Answer from the drawing. Dimensions are ordinates in mm from the lowest x, y and z of the part. Coordinates: 2 decimals unless noted, no trailing zeros. Order: outer loops, then holes, each group sorted by start corner. A loop starts at its lowest first (then second) coordinate and runs counter-clockwise, first axis right, second up. Notation, with made-up numbers: (15.25, -26.5) -> (25.25, -26.5) arc R17 ccw to (25.25, 1.5) -> close; hole circle Ø1 at (75, -26.5). An arc over 180 degrees is marked (long way). Answer as a JSON object with one key per item and string values. Group by question number.
1) Section B-B on x = 10.25 is taken. Determine the outline of the cut face in (y, z).
2) Section A-A on y = 31.75 is taken. Determine the outline of the cut face in (x, z).
3) Consider L1, parallel to X at y = 31.75, z = 1.25; L2, parallel to Y at x = 12.7, z = 0.6; L3, parallel to Y at x = 6.25, z = 0.8. Determine where each line is inside the solid, lowest interval first.
4) Section D-D on y = 40 is taken. Determine the outline of the cut face in (x, z).
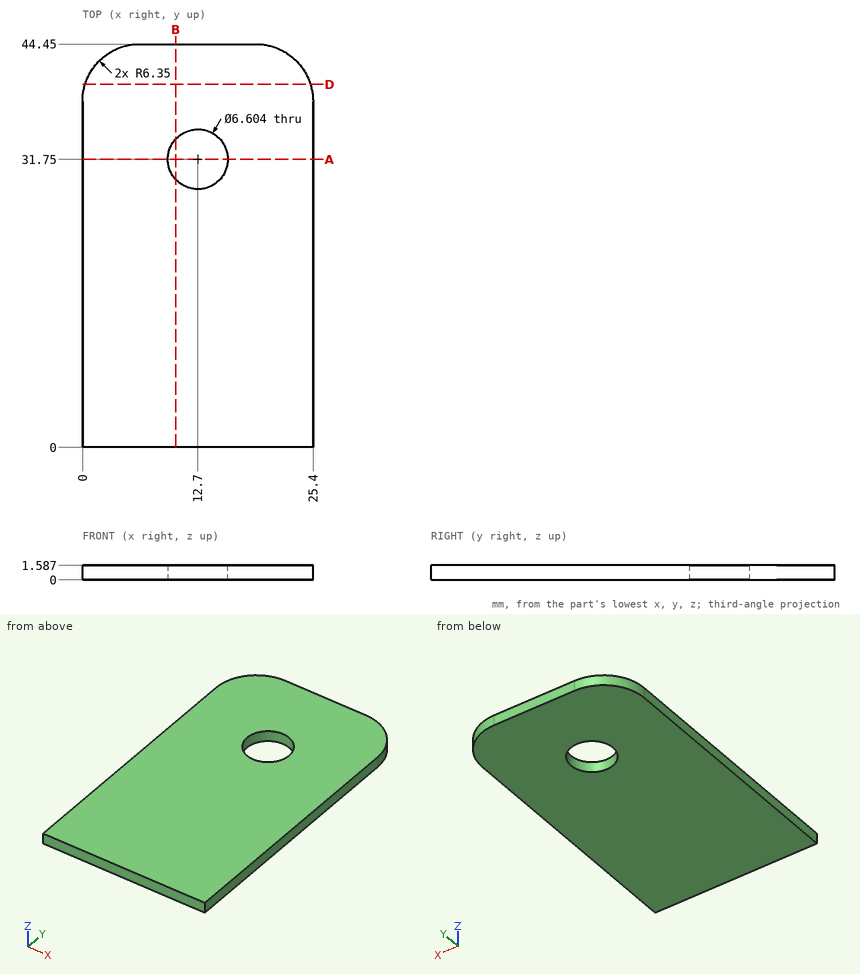
Worked answers:
{
 "1": {"outline": "(0, 0) -> (29.54, 0) -> (29.54, 1.59) -> (0, 1.59) -> close; (33.96, 0) -> (44.45, 0) -> (44.45, 1.59) -> (33.96, 1.59) -> close"},
 "2": {"outline": "(0, 0) -> (9.4, 0) -> (9.4, 1.59) -> (0, 1.59) -> close; (16, 0) -> (25.4, 0) -> (25.4, 1.59) -> (16, 1.59) -> close"},
 "3": {"L1": "x = 0 to 9.4, 16 to 25.4", "L2": "y = 0 to 28.45, 35.05 to 44.45", "L3": "y = 0 to 44.45"},
 "4": {"outline": "(0.29, 0) -> (25.11, 0) -> (25.11, 1.59) -> (0.29, 1.59) -> close"}
}
